Source: CAD feature listing. Evaluate the final solid. Frame: model axes, mm. A direction names the side the tool comes from. Round coordinates to 2 decimals unless told otherwise and drop trailing zeros. Order: outer loops, then holes, each group sorted by start corner. A loop starts at its lowest first (then second) coordinate and runs counter-clockwise, first axis right, second up. Notation, with made-up numbers: (48.25, 15.25) - (80.25, 15.25) arc R10 ccw to (80.25, 30.25) - close; hole circle Ø7 at (59, -19.75). An arc over 180 degrees is marked (long way). Use one line per item in the form item = value. Start each with the question number.
Q1. Cut plane A-A, the plane x = 31.5. Return the cut outline in (y, z).
Q2. Pin query (flat end, axial travel): pin 1 Ø8 at (x, y) = (24.5, -6) entering from -Z; pin 2 Ø1 at (x, y) = (-43, 43) entering from +Z. Return the tip coordinate at first contact, or that it passes through.
Q3. Cut plane B-B, the plane y = -14.5. Return the cut outline in (x, z).
Q4. Cut plane D-D, the plane y = 21. Return the cut outline in (x, z), and give its area (4 significant figures).
Q5. Cut plane C-C, the plane z = -1.2. Return the cut outline in (x, y).
Q6. Draft query along X for faces 1 (the flat face through (-1, 11, 1.5)), 2 (the cylindrical face through (-44.43, -44.4, 0.76)), 3 (the cylindrical face through (-38.244, 6.725, 0.74)). Return one class per face: released by +X, released by -X, zero draft, split by the parting line, or undercut.
Q7. Ray query, line 1 (Y direction, x = 28, z = -0.05); line 2 (Y direction, x = 42.25, z = 0.85). Return the intervals inside material, ascending. Write a range as [from, to].
Q8. Set-up query: faces 4 (the flat face through (44, 4.25, -1)), 5 (the cylindrical face through (-44.4, 44.43, 0.76)), 6 (the cylindrical face through (41.034, -41.135, 0.76)), 7 (the flat face through (42.25, 28, -1)). Return all of +Z, -Z, +X, -X, +Y, -Y with unobstructed straight access to the full face (end or side cutting, diameter ignored); none if empty.
Autodesk Inventor part; units mm, degrees
ref_plane "YZ Plane" through (0, 0, 0) normal (1, 0, 0) x (0, 1, 0)
ref_plane "XZ Plane" through (0, 0, 0) normal (0, 1, 0) x (-1, 0, 0)
ref_plane "XY Plane" through (0, 0, 0) normal (0, 0, 1) x (1, 0, 0)
sketch "Sketch1" plane through (0, 0, 0) normal (0, 0, 1) x (1, 0, 0)
  arc A0 (-45, -43.5) -> (-43.5, -45) centre (-43.5, -43.5) ccw
  line L0 (-43.5, -45) -> (43.5, -45)
  arc A1 (43.5, -45) -> (45, -43.5) centre (43.5, -43.5) ccw
  line L1 (45, -43.5) -> (45, 4.25)
  line L2 (45, 4.25) -> (42.25, 4.25)
  line L3 (42.25, 4.25) -> (42.25, -40.75)
  arc A2 (40.75, -42.25) -> (42.25, -40.75) centre (42.25, -42.25) ccw
  line L4 (40.75, -42.25) -> (-40.75, -42.25)
  arc A3 (-42.25, -40.75) -> (-40.75, -42.25) centre (-42.25, -42.25) ccw
  line L5 (-42.25, -40.75) -> (-42.25, 40.75)
  arc A4 (-40.75, 42.25) -> (-42.25, 40.75) centre (-42.25, 42.25) ccw
  line L6 (-40.75, 42.25) -> (-5, 42.25)
  line L7 (-5, 42.25) -> (-5, 45)
  line L8 (-5, 45) -> (-43.5, 45)
  arc A5 (-43.5, 45) -> (-45, 43.5) centre (-43.5, 43.5) ccw
  line L9 (-45, 43.5) -> (-45, -43.5)
  line L10 (-45, 45) -> (45, 45)
  line L11 (45, 45) -> (45, -45)
  line L12 (45, -45) -> (-45, -45)
  line L13 (-45, -45) -> (-45, 45)
  line L14 (-45, 45) -> (45, -45) construction
  line L15 (45, 45) -> (-45, -45) construction
  line L16 (37.25, -9.75) -> (-34.75, -9.75)
  line L17 (-34.75, -9.75) -> (-34.75, -34.75)
  line L18 (-34.75, -34.75) -> (37.25, -34.75)
  line L19 (37.25, -34.75) -> (37.25, -9.75)
  circle A6 centre (-32, 7) radius 6.25
  point P0 (0, 0)
  dimension "d0" = 90
  dimension "d1" = 90
  dimension "d2" = 72
  dimension "d3" = 25
  dimension "d4" = 7.5
  dimension "d5" = 5
  dimension "d6" = 12.5
  dimension "d19" = 38
  dimension "d20" = 13
extrude "Extrusion1" add sketch "Sketch1" along normal blind 1.5
fillet "Fillet1" radius 2 4 edges at (45, -45, 0.75) (-45, -45, 0.75) (-45, 45, 0.75) (45, 45, 0.75)
sketch "Sketch2" plane through (0, 0, 1.5) normal (0, 0, 1) x (1, 0, 0)
  arc A0 (40.75, -42.25) -> (42.25, -40.75) centre (42.25, -42.25) ccw
  arc A1 (-42.25, -40.75) -> (-40.75, -42.25) centre (-42.25, -42.25) ccw
  arc A2 (-40.75, 42.25) -> (-42.25, 40.75) centre (-42.25, 42.25) ccw
  arc A3 (42.25, 40.75) -> (40.75, 42.25) centre (42.25, 42.25) ccw
  circle A4 centre (42.25, 42.25) radius 1.65
  circle A5 centre (-42.25, 42.25) radius 1.65
  circle A6 centre (-42.25, -42.25) radius 1.65
  circle A7 centre (42.25, -42.25) radius 1.65
  point P0 (0, 0)
  dimension "d12" = 3.3
  dimension "d13" = 3.3
  dimension "d14" = 3.3
  dimension "d15" = 3.3
extrude "Extrusion2" cut sketch "Sketch2" against normal blind 3
sketch "Sketch3" plane through (0, 0, 0) normal (0, 0, -1) x (-1, 0, 0)
  arc A0 (43.5, -45) -> (45, -43.5) centre (43.5, -43.5) ccw
  line L0 (43.5, -45) -> (-43.5, -45)
  arc A1 (-45, -43.5) -> (-43.5, -45) centre (-43.5, -43.5) ccw
  line L1 (-45, -43.5) -> (-45, 4.25)
  line L2 (-45, 4.25) -> (-42.25, 4.25)
  line L3 (-42.25, 4.25) -> (-42.25, -40.75)
  arc A2 (-42.25, -40.75) -> (-40.75, -42.25) centre (-42.25, -42.25) ccw
  line L4 (-40.75, -42.25) -> (40.75, -42.25)
  arc A3 (40.75, -42.25) -> (42.25, -40.75) centre (42.25, -42.25) ccw
  line L5 (42.25, -40.75) -> (42.25, 40.75)
  arc A4 (42.25, 40.75) -> (40.75, 42.25) centre (42.25, 42.25) ccw
  line L6 (40.75, 42.25) -> (5, 42.25)
  line L7 (5, 42.25) -> (5, 45)
  line L8 (5, 45) -> (43.5, 45)
  arc A5 (45, 43.5) -> (43.5, 45) centre (43.5, 43.5) ccw
  line L9 (45, 43.5) -> (45, -43.5)
  arc A6 (-43.5, 45) -> (-45, 43.5) centre (-43.5, 43.5) ccw
  line L10 (-43.5, 45) -> (-5, 45)
  line L11 (-5, 45) -> (-5, 42.25)
  line L12 (-5, 42.25) -> (-40.75, 42.25)
  arc A7 (-40.75, 42.25) -> (-42.25, 40.75) centre (-42.25, 42.25) ccw
  line L13 (-42.25, 40.75) -> (-42.25, 15.75)
  line L14 (-42.25, 15.75) -> (-45, 15.75)
  line L15 (-45, 15.75) -> (-45, 43.5)
  point P0 (0, 0)
extrude "Extrusion3" add sketch "Sketch3" along normal blind 3
properties part number "covor"
Completed:
q1.outline = (-45, -3) - (-42.25, -3) - (-42.25, 0) - (-34.75, 0) - (-34.75, 1.5) - (-45, 1.5) - close; (-9.75, 0) - (42.25, 0) - (42.25, -3) - (45, -3) - (45, 1.5) - (-9.75, 1.5) - close
q2.pin_1 = 0
q2.pin_2 = 0
q3.outline = (-45, -3) - (-42.25, -3) - (-42.25, 0) - (-34.75, 0) - (-34.75, 1.5) - (-45, 1.5) - close; (37.25, 0) - (42.25, 0) - (42.25, -3) - (45, -3) - (45, 1.5) - (37.25, 1.5) - close
q4.outline = (-45, -3) - (-42.25, -3) - (-42.25, 0) - (42.25, 0) - (42.25, -3) - (45, -3) - (45, 1.5) - (-45, 1.5) - close
q4.area = 151.5 mm2
q5.outline = (-45, -43.5) arc R1.5 ccw to (-43.5, -45) - (43.5, -45) arc R1.5 ccw to (45, -43.5) - (45, 4.25) - (42.25, 4.25) - (42.25, -40.75) arc R1.5 cw (long way) to (40.75, -42.25) - (-40.75, -42.25) arc R1.5 cw (long way) to (-42.25, -40.75) - (-42.25, 40.75) arc R1.5 cw (long way) to (-40.75, 42.25) - (-5, 42.25) - (-5, 45) - (-43.5, 45) arc R1.5 ccw to (-45, 43.5) - close; (5, 42.25) - (40.75, 42.25) arc R1.5 cw (long way) to (42.25, 40.75) - (42.25, 15.75) - (45, 15.75) - (45, 43.5) arc R1.5 ccw to (43.5, 45) - (5, 45) - close
q6.face_1 = zero draft
q6.face_2 = released by -X
q6.face_3 = undercut
q7.line_1 = [-45, -42.25], [42.25, 45]
q7.line_2 = [-45, -43.9], [-40.6, 40.6], [43.9, 45]
q8.face_4 = -Z, +X
q8.face_5 = +Z, -X, +Y
q8.face_6 = +Z
q8.face_7 = -Z
